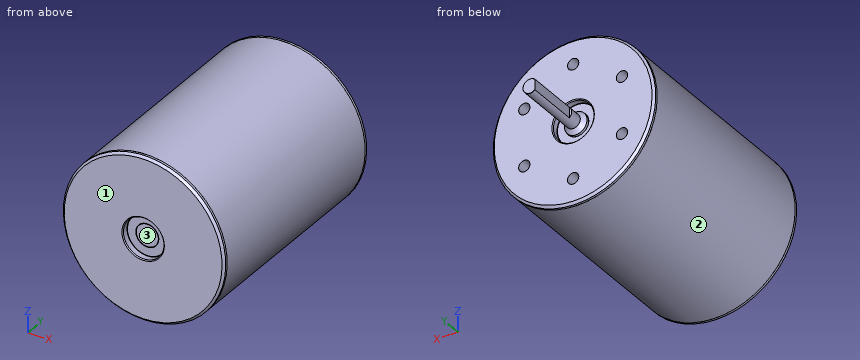
```python
from build123d import *

# Parameters (mm, degrees)
ESQUISSE2_W                  = 0.5
ESQUISSE2_H                  = 2.313006702
ENL_V_MAT_EXTRU_1_DEPTH      = 12
R_P_TITION_CIRCULAIRE1_COUNT = 6


with BuildPart() as part:
    # Esquisse1 → Révolution1 (revolve)
    with BuildSketch(Plane.XY, mode=Mode.PRIVATE) as r_volution1_sk:
        Polygon((0, 65), (-1.5375, 65), (-1.5875, 64.95), (-1.5875, 50), (-2.5, 49.0875), (-2.5, 48.5), (-2.55, 48.55), (-4.4, 48.55), (-4.45, 48.5), (-4.5, 48.55), (-4.5, 49.8), (-4.7, 50), (-17.5, 50), (-18, 49.5), (-18, 49), (-17.995, 48.995), (-18, 48.99), (-18, 1.01), (-17.995, 1.005), (-18, 1), (-18, 0.5), (-17.5, 0), (-4.7, 0), (-4.5, 0.2), (-4.5, 1.45), (-4.45, 1.5), (-4.4, 1.45), (-2.55, 1.45), (-2.5, 1.5), (-2.45, 1.45), (0, 1.45), align=None)
    revolve(r_volution1_sk.sketch.rotate(Axis((0, -4.92112906, 0), (0, 1, 0)), 270), axis=Axis((0, -4.92112906, 0), (0, 1, 0)))

    # Esquisse2 → Enlèv. mat.-Extru.1 (cut)
    with BuildSketch(Plane(origin=(0, 65, 0), x_dir=(1, 0, 0), z_dir=(0, 1, 0))):
        with Locations((-1.3375, 0)):
            Rectangle(ESQUISSE2_W, ESQUISSE2_H)
    extrude(amount=-ENL_V_MAT_EXTRU_1_DEPTH, mode=Mode.SUBTRACT)

    # Esquisse4 → Trou taraudé M31 (revolve, cut)
    with BuildSketch(Plane(origin=(0, 50, -12.5), x_dir=(0, 0, 1), z_dir=(1, 0, 0))):
        Polygon((0, 0), (0, 7.751075774), (1.25, 7), (1.25, 0), align=None)
    trou_taraud_m31 = revolve(axis=Axis((0, 56.35, -12.5), (0, -1, 0)), mode=Mode.SUBTRACT)

    # Répétition circulaire1: Trou taraudé M31 ×6 about axis
    r_p_tition_circulaire1_axis = Axis((0, 0, 0), (0, 1, 0))
    for i in range(1, R_P_TITION_CIRCULAIRE1_COUNT):
        add(trou_taraud_m31.rotate(r_p_tition_circulaire1_axis, i * 360 / R_P_TITION_CIRCULAIRE1_COUNT), mode=Mode.SUBTRACT)


solid = part.part
```
The listing builds one solid part. Answer for the finished solid, in the listing's coordinates (mm). Face numbers are marked on the shaded views. Give positions to 0.01 mm unless a question says otherwise; leave off trailing zeros. Order: outer loops, then holes, each group sorted by start corner. A loop starts at its lowest first (then second) coordinate and runs counter-clockwise, first axis right, second up.
Item 1: The part is cut by section A-A, the plane y = 33. Give the vertices of the cut face in (x, z).
From the geometry:
outline: circle Ø36 at (0, 0)
Item 2: Given pin 1 Ø10 at (y, z) = (52, -13.5) entering from +X; pin 2 Ø2.5 at (x, z) = (0.5, 1) entering from -Y; pin 3 Ø1.2 at (y, z) = (59.5, -0.5) entering from -X; pin 4 Ø2 at (x, z) = (-10.83, -6.25) entering from -Y, each flat-ended and moving along its own axis, determine where each tip first touches the part or whether it passes through.
From the geometry:
pin 1: stops at x = 15.49
pin 2: stops at y = 1.45
pin 3: stops at x = -1.09
pin 4: stops at y = 0
Item 3: For a pull along Z with two mould halves and no side action, classify the marked faces 1, 2 and 3 as pulls with the +Z half, pulls with the -Z half, needs draft (parallel to the pull), parting line crosses it, or undercut.
From the geometry:
face 1: needs draft
face 2: parting line crosses it
face 3: undercut
Item 4: Find the intervals of material crossed by probe 1 along X at (y, z) = (45.5, -6.25); probe 2 along Y at (x, z) = (-2, -10); probe 3 along Z at (x, y) = (-0.5, 37.5), in increasing order.
From the geometry:
probe 1: x = -16.88 to -12.08, -9.58 to 9.58, 12.08 to 16.88
probe 2: y = 0 to 50
probe 3: z = -17.99 to 17.99
